Check sheet for the modelled part. Datum: model origin and axes. Units: mm. A direction names the side the tool comes from. Give positions to 0.01 mm unless a question says otherwise; leave off trailing zeros. Write each question's results on one line, items separated by ' | '. Start each with the question number.
1. Material ranges on line 1 along X through (y, z) = (-4, 11.5) (3 decimals); line 2 along X through (y, z) = (-5, 12.5) (3 decimals); line 3 along X through (y, z) = (-2.5, 3.5) (3 decimals), recorded low to high.
2. Go/stop test with flat-tipped pins: pin 1 (1.9 mm diameter, centred on y = 2, z = 11.5, fed in from +X); pin 2 (5.5 mm diameter, centred on x = 0, z = 13, fed in from +Y). Record where each tip stops, or that it passes through.
3. Draft check along Z on faces 3 (the flat face through (-6.35, -2, 7)), 4 (the conical face through (-2.593, 4.484, -0.589)), 5 (the flat face through (-5.57, -4, 15.07)). Enter one of: pulls with the +Z half, pulls with the -Z half, needs draft (parallel to the pull), parting line crosses it, or undercut.
4. Tool access check on faces 1 (the flat face through (13.47, -1.05, 8.8)), 2 (the flat face through (11.96, 2.33, 5.76)). Record the directions out of +Z, -Z, +X, -X, +Y, -Y that give a thin tool (end or side, any length) a straight path to the whole face; none if there is none.
5. Sectioned sample at B-B on y = 0. Give the number of separate pieces and of enclosed holes in the cut face, and give its area (3 significant figures).
```python
from build123d import *

# Parameters (mm, degrees)
SKETCH1_W               = 12.7
SKETCH1_H               = 12.7
BOSS_EXTRUDE1_DEPTH     = 6.35
SKETCH2_W               = 22.225
SKETCH2_H               = 9.525
BOSS_EXTRUDE2_DEPTH     = 4.7625
CHAMFER1_START          = -6.35
CHAMFER1_DEPTH          = 12.7
CUT_EXTRUDE1_DEPTH      = 7.9375
F_6_CLEARANCE_HOLE1_D   = 4.3053
CHAMFER3_SIZE           = 9.525
F_1_4_CLEARANCE_HOLE1_D = 7.14248
CUT_EXTRUDE2_DEPTH      = 9.525
CUT_EXTRUDE3_DEPTH      = 26.793821935


with BuildPart() as part:
    # Sketch1 → Boss-Extrude1 (new, symmetric)
    with BuildSketch(Plane(origin=(0, 0, 0), x_dir=(1, 0, 0), z_dir=(0, 1, 0))):
        Rectangle(SKETCH1_W, SKETCH1_H)
    extrude(amount=BOSS_EXTRUDE1_DEPTH, both=True)

    # Sketch2 → Boss-Extrude2 (add)
    with BuildSketch(Plane.XZ.offset(6.35)):
        with Locations((4.7625, 11.1125)):
            Rectangle(SKETCH2_W, SKETCH2_H)
    extrude(amount=-BOSS_EXTRUDE2_DEPTH)

    # Chamfer1: read off the stored shape, not the designer's step
    # Chamfer1 outline → Chamfer1 (add)
    with BuildSketch(Plane(origin=(0, 0, 0), x_dir=(1, 0, 0), z_dir=(0, 1, 0)).offset(CHAMFER1_START)):
        Polygon((15.875, -6.35), (6.35, 3.175), (6.35, -6.35), align=None)
    extrude(amount=CHAMFER1_DEPTH)

    # Sketch3 → Cut-Extrude1 (cut)
    with BuildSketch(Plane(origin=(0, 6.35, 0), x_dir=(1, 0, 0), z_dir=(0, 1, 0))):
        Polygon((6.35, 3.175), (6.35, -6.35), (15.875, -6.35), align=None)
    extrude(amount=-CUT_EXTRUDE1_DEPTH, mode=Mode.SUBTRACT)

    # #6 Clearance Hole1 (through all)
    with Locations(Plane(origin=(0, -1.5875, 0), x_dir=(1, 0, 0), z_dir=(0, 1, 0))):
        with Locations((-1.5875, -11.1125), (11.1125, -11.1125)):
            Hole(F_6_CLEARANCE_HOLE1_D / 2)

    # Chamfer3
    # the kernel refuses this chamfer: 9.525 mm, written as the material it adds along each edge
    with BuildSketch(Plane(origin=(6.35, -1.5875, -27.67028046), x_dir=(1, 0, 0), z_dir=(0, 0, 1))) as chamfer3_piece_1_section:
        Polygon((CHAMFER3_SIZE, 0), (0, CHAMFER3_SIZE), (0, 0), align=None)
    chamfer3_piece_1 = extrude(amount=34.02028046, mode=Mode.PRIVATE)
    chamfer3_piece_1 = split(chamfer3_piece_1, bisect_by=Plane(origin=(6.35, 6.35, -27.67028046), z_dir=(0, -1, 0)), keep=Keep.TOP, mode=Mode.PRIVATE)
    chamfer3_piece_1 = split(chamfer3_piece_1, bisect_by=Plane(origin=(-5.89764023, -1.5875, -15.42264023), z_dir=(-0.7071067811865475, 0, 0.7071067811865476)), keep=Keep.TOP, mode=Mode.PRIVATE)
    add(chamfer3_piece_1)
    with BuildSketch(Plane(origin=(-6.35, -1.5875, 6.35), x_dir=(0, 1, 0), z_dir=(1, 0, 0))) as chamfer3_piece_2_section:
        Polygon((CHAMFER3_SIZE, 0), (0, CHAMFER3_SIZE), (0, 0), align=None)
    chamfer3_piece_2 = extrude(amount=12.7, mode=Mode.PRIVATE)
    chamfer3_piece_2 = split(chamfer3_piece_2, bisect_by=Plane(origin=(-6.35, 6.35, 6.35), z_dir=(0, -1, 0)), keep=Keep.TOP, mode=Mode.PRIVATE)
    chamfer3_piece_2 = chamfer3_piece_2 - Plane(origin=(-1.5875, -1.5875, 11.1125), x_dir=(-1, 0, 0), z_dir=(0, -1, 0)) * Cylinder(2.15265, 64, mode=Mode.PRIVATE)
    add(chamfer3_piece_2)
    with BuildSketch(Plane(origin=(-6.35, -1.5875, 6.35), x_dir=(0, 1, 0), z_dir=(1, 0, 0))) as chamfer3_piece_3a_section:
        Polygon((CHAMFER3_SIZE, 0), (0, CHAMFER3_SIZE), (0, 0), align=None)
    chamfer3_piece_3a = extrude(amount=37.19528046, mode=Mode.PRIVATE)
    chamfer3_piece_3a = split(chamfer3_piece_3a, bisect_by=Plane(origin=(-6.35, 6.35, 6.35), z_dir=(0, -1, 0)), keep=Keep.TOP, mode=Mode.PRIVATE)
    chamfer3_piece_3a = split(chamfer3_piece_3a, bisect_by=Plane(origin=(6.35, -1.5875, 6.35), z_dir=(1, 0, 0)), keep=Keep.TOP, mode=Mode.PRIVATE)
    chamfer3_piece_3a = split(chamfer3_piece_3a, bisect_by=Plane(origin=(15.875, -1.5875, 6.35), z_dir=(-1, 0, 0)), keep=Keep.TOP, mode=Mode.PRIVATE)
    chamfer3_piece_3a = chamfer3_piece_3a - Plane(origin=(11.1125, -1.5875, 11.1125), x_dir=(-1, 0, 0), z_dir=(0, -1, 0)) * Cylinder(2.15265, 113, mode=Mode.PRIVATE)
    with BuildSketch(Plane(origin=(6.35, -1.5875, -27.67028046), x_dir=(1, 0, 0), z_dir=(0, 0, 1))) as chamfer3_piece_3b_section:
        Polygon((CHAMFER3_SIZE, 0), (0, CHAMFER3_SIZE), (0, 0), align=None)
    chamfer3_piece_3b = extrude(amount=58.515560921, mode=Mode.PRIVATE)
    chamfer3_piece_3b = split(chamfer3_piece_3b, bisect_by=Plane(origin=(6.35, -1.5875, 6.35), z_dir=(0, 0, 1)), keep=Keep.TOP, mode=Mode.PRIVATE)
    chamfer3_piece_3b = split(chamfer3_piece_3b, bisect_by=Plane(origin=(6.35, 6.35, -27.67028046), z_dir=(0, -1, 0)), keep=Keep.TOP, mode=Mode.PRIVATE)
    chamfer3_piece_3b = split(chamfer3_piece_3b, bisect_by=Plane(origin=(6.35, -1.5875, 15.875), z_dir=(0, 0, -1)), keep=Keep.TOP, mode=Mode.PRIVATE)
    chamfer3_piece_3b = chamfer3_piece_3b - Plane(origin=(11.1125, -1.5875, 11.1125), x_dir=(-1, 0, 0), z_dir=(0, -1, 0)) * Cylinder(2.15265, 156, mode=Mode.PRIVATE)
    chamfer3_piece_3 = chamfer3_piece_3a & chamfer3_piece_3b
    add(chamfer3_piece_3)

    # Sketch9 → Hole1 (revolve, cut)
    with BuildSketch(Plane(origin=(-6.35, 0, 0), x_dir=(0, 0, 1), z_dir=(0, 1, 0))):
        Polygon((0, 0), (0, 7.62), (4.4323, 7.62), (4.6101, 0), align=None)
    revolve(axis=Axis((103.65, 0, 0), (-1, 0, 0)), mode=Mode.SUBTRACT)

    # 1/4 Clearance Hole1 (through all)
    with Locations(Plane.ZY.offset(6.35)):
        with Locations((0, 0)):
            Hole(F_1_4_CLEARANCE_HOLE1_D / 2)

    # Sketch12 → Cut-Extrude2 (cut)
    with BuildSketch(Plane(origin=(0, 6.35, 0), x_dir=(1, 0, 0), z_dir=(0, 1, 0))):
        Polygon((-4.8895, -9.206089411), (-4.8895, -13.018910589), (-1.5875, -14.925321178), (1.7145, -13.018910589), (1.7145, -9.206089411), (-1.5875, -7.299678822), align=None)
        Polygon((8.41642829, -8.41642829), (7.429597553, -12.099330736), (10.125669264, -14.795402447), (13.80857171, -13.80857171), (14.795402447, -10.125669264), (12.099330736, -7.429597553), align=None)
    extrude(amount=-CUT_EXTRUDE2_DEPTH, mode=Mode.SUBTRACT)

    # Sketch15 → Cut-Extrude3 (cut, through all)
    with BuildSketch(Plane(origin=(0, 6.35, 0), x_dir=(1, 0, 0), z_dir=(0, 1, 0))):
        Polygon((6.35, 3.175), (3.175, 6.35), (6.35, 6.35), align=None)
    extrude(amount=-CUT_EXTRUDE3_DEPTH, mode=Mode.SUBTRACT)

    # Chamfer4
    # the kernel refuses this chamfer: 1.5875 mm, written as the material it takes off along each edge
    with BuildSketch(Plane(origin=(-5.291666667, 5.291666667, -5.291666667), x_dir=(0.7071067811865476, 0.7071067811865476, 0), z_dir=(-0.5773502691896257, 0.577350269189626, -0.5773502691896257))) as chamfer4_piece_1:
        Polygon((-1.122532015, -0.648094161), (1.122532015, -0.648094161), (0, 1.296188322), align=None)
    extrude(amount=2.016395815, mode=Mode.SUBTRACT)
    with BuildSketch(Plane(origin=(15.875, -10.432546743, 15.875), x_dir=(0, 0, -1), z_dir=(0, 1, 0))) as chamfer4_piece_2:
        with BuildLine():
            Line((1.632401281, -0.044901281), (-0.044901281, 1.632401281))
            Line((-0.044901281, 1.632401281), (-0.076651281, 1.632401281))
            ThreePointArc((-0.076651281, 1.632401281), (-0.03175, 0.81620064), (-0.03175, 0))
            Line((-0.03175, 0), (0, -0.03175))
            ThreePointArc((0, -0.03175), (0.81620064, -0.03175), (1.632401281, -0.076651281))
            Line((1.632401281, -0.076651281), (1.632401281, -0.044901281))
        make_face()
    extrude(amount=12.927593487, mode=Mode.SUBTRACT)
    with BuildSketch(Plane(origin=(-10.432546743, 6.35, -6.35), x_dir=(0, -1, 0), z_dir=(1, 0, 0))) as chamfer4_piece_3:
        with BuildLine():
            Line((1.632401281, 0.044901281), (-0.044901281, -1.632401281))
            Line((-0.044901281, -1.632401281), (-0.076651281, -1.632401281))
            ThreePointArc((-0.076651281, -1.632401281), (-0.03175, -0.81620064), (-0.03175, 0))
            Line((-0.03175, 0), (0, 0.03175))
            ThreePointArc((0, 0.03175), (0.81620064, 0.03175), (1.632401281, 0.076651281))
            Line((1.632401281, 0.076651281), (1.632401281, 0.044901281))
        make_face()
    extrude(amount=17.690093487, mode=Mode.SUBTRACT)
    with BuildSketch(Plane(origin=(-6.35, -10.432546743, 15.875), x_dir=(0, 0, -1), z_dir=(0, 1, 0))) as chamfer4_piece_4:
        with BuildLine():
            Line((1.632401281, 0.044901281), (-0.044901281, -1.632401281))
            Line((-0.044901281, -1.632401281), (-0.076651281, -1.632401281))
            ThreePointArc((-0.076651281, -1.632401281), (-0.03175, -0.81620064), (-0.03175, 0))
            Line((-0.03175, 0), (0, 0.03175))
            ThreePointArc((0, 0.03175), (0.81620064, 0.03175), (1.632401281, 0.076651281))
            Line((1.632401281, 0.076651281), (1.632401281, 0.044901281))
        make_face()
    extrude(amount=12.927593487, mode=Mode.SUBTRACT)
    with BuildSketch(Plane(origin=(-6.35, 9.236796487, 5.050703513), x_dir=(1, 0, 0), z_dir=(0, -0.7071067811865476, 0.7071067811865476))) as chamfer4_piece_5:
        with BuildLine():
            Line((1.632401281, 0.044901281), (-0.044901281, -1.632401281))
            Line((-0.044901281, -1.632401281), (-0.076651281, -1.632401281))
            ThreePointArc((-0.076651281, -1.632401281), (-0.03175, -0.81620064), (-0.03175, 0))
            Line((-0.03175, 0), (0, 0.03175))
            ThreePointArc((0, 0.03175), (0.81620064, 0.03175), (1.632401281, 0.076651281))
            Line((1.632401281, 0.076651281), (1.632401281, 0.044901281))
        make_face()
    extrude(amount=19.390413638, mode=Mode.SUBTRACT)
    with BuildSketch(Plane(origin=(-6.35, 6.35, 12.020046743), x_dir=(0, -1, 0), z_dir=(0, 0, -1))) as chamfer4_piece_6:
        with BuildLine():
            Line((1.632401281, 0.044901281), (-0.044901281, -1.632401281))
            Line((-0.044901281, -1.632401281), (-0.076651281, -1.632401281))
            ThreePointArc((-0.076651281, -1.632401281), (-0.03175, -0.81620064), (-0.03175, 0))
            Line((-0.03175, 0), (0, 0.03175))
            ThreePointArc((0, 0.03175), (0.81620064, 0.03175), (1.632401281, 0.076651281))
            Line((1.632401281, 0.076651281), (1.632401281, 0.044901281))
        make_face()
    extrude(amount=22.452593487, mode=Mode.SUBTRACT)
    with BuildSketch(Plane(origin=(-6.35, 10.432546743, -6.35), x_dir=(0, 0, 1), z_dir=(0, -1, 0))) as chamfer4_piece_7:
        with BuildLine():
            Line((1.632401281, 0.044901281), (-0.044901281, -1.632401281))
            Line((-0.044901281, -1.632401281), (-0.076651281, -1.632401281))
            ThreePointArc((-0.076651281, -1.632401281), (-0.03175, -0.81620064), (-0.03175, 0))
            Line((-0.03175, 0), (0, 0.03175))
            ThreePointArc((0, 0.03175), (0.81620064, 0.03175), (1.632401281, 0.076651281))
            Line((1.632401281, 0.076651281), (1.632401281, 0.044901281))
        make_face()
    extrude(amount=20.865093487, mode=Mode.SUBTRACT)
    with BuildSketch(Plane(origin=(10.824296487, 6.35, 1.299296487), x_dir=(0, -1, 0), z_dir=(-0.7071067811865507, 0, -0.7071067811865444))) as chamfer4_piece_8:
        with BuildLine():
            Line((1.632401281, -0.044901281), (-0.044901281, 1.632401281))
            Line((-0.044901281, 1.632401281), (-0.076651281, 1.632401281))
            ThreePointArc((-0.076651281, 1.632401281), (-0.03175, 0.81620064), (-0.03175, 0))
            Line((-0.03175, 0), (0, -0.03175))
            ThreePointArc((0, -0.03175), (0.81620064, -0.03175), (1.632401281, -0.076651281))
            Line((1.632401281, -0.076651281), (1.632401281, -0.044901281))
        make_face()
    extrude(amount=14.900285578, mode=Mode.SUBTRACT)


solid = part.part
```
Output values:
1) line 1: -6.35 to -3.705, 0.53 to 8.995, 13.23 to 15.875 | line 2: -6.35 to -3.233, 0.058 to 9.467, 12.758 to 15.875 | line 3: 1.27 to 13.025
2) pin 1: x = 7.84 | pin 2: y = 3.44
3) face 3: needs draft | face 4: undercut | face 5: pulls with the +Z half
4) face 1: +Y | face 2: +Z, -Z, +X, +Y
5) separate pieces: 3 | enclosed holes: 0 | area: 160 mm2
